Read the model definition and answer for the solid it produces. Units are mm, in the model's axes. A direction names the side the tool comes from. Give positions to 0.01 mm unless a question says otherwise; leave off trailing zeros. Loops run counter-clockwise (first coordinate to the right, second up) from the corner with the lowest first, then second, coordinate; pieces in that order, holes last. Notation, with made-up numbers: (53.25, 89.5) -> (112.25, 89.5) arc R24 cw to (112.25, 119.5) -> close; hole circle Ø5 at (21.25, 41). An arc over 180 degrees is marked (long way). Return JSON: item names as keys, results as strings. Group by question number.
from build123d import *

# Parameters (mm, degrees)
SKETCH1_W               = 228.6
SKETCH1_H               = 228.6
BOSS_EXTRUDE1_DEPTH     = 67
SKETCH2_W               = 35.766
SKETCH2_H               = 35.766
CUT_EXTRUDE1_DEPTH      = 76.2
CUT_EXTRUDE3_DEPTH      = 4
CUT_EXTRUDE3_DEPTH_BACK = 4
SKETCH4_W               = 67
SKETCH4_H               = 35.766
CUT_EXTRUDE4_DEPTH      = 4
CUT_EXTRUDE4_DEPTH_BACK = 4
SKETCH5_W               = 67
SKETCH5_H               = 37.77
SKETCH5_H_2             = 35.766
CUT_EXTRUDE5_DEPTH      = 4
CUT_EXTRUDE5_DEPTH_BACK = 4
SKETCH6_W               = 67
SKETCH6_H               = 35.766
SKETCH6_H_2             = 37.77
CUT_EXTRUDE6_DEPTH      = 4
CUT_EXTRUDE6_DEPTH_BACK = 4
SKETCH9_W               = 67
SKETCH9_H               = 37.766
SKETCH9_H_2             = 35.766
SKETCH9_H_3             = 37.77
SKETCH10_W              = 67
SKETCH10_H              = 2
CUT_EXTRUDE7_DEPTH      = 233.316821509
SKETCH11_W              = 67
SKETCH11_H              = 2
CUT_EXTRUDE8_DEPTH      = 231.673489808


with BuildPart() as part:
    # Sketch1 → Boss-Extrude1 (new body)
    with BuildSketch(Plane(origin=(0, 0, 0), x_dir=(0, 0, -1), z_dir=(1, 0, 0))):
        Rectangle(SKETCH1_W, SKETCH1_H)
    extrude(amount=BOSS_EXTRUDE1_DEPTH)

    # Sketch2 → Cut-Extrude1 (cut)
    with BuildSketch(Plane(origin=(67, 0, 0), x_dir=(0, 0, -1), z_dir=(1, 0, 0))):
        with Locations((-94.417, 94.417)):
            Rectangle(SKETCH2_W, SKETCH2_H)
        with Locations((-56.651, 94.417)):
            Rectangle(SKETCH2_W, SKETCH2_H)
        with Locations((18.881, 94.417)):
            Rectangle(SKETCH2_W, SKETCH2_H)
        with Locations((-18.885, 94.417)):
            Rectangle(SKETCH2_W, SKETCH2_H)
        with Locations((56.647, 94.417)):
            Rectangle(SKETCH2_W, SKETCH2_H)
        with Locations((94.413, 94.417)):
            Rectangle(SKETCH2_W, SKETCH2_H)
        with Locations((56.647, 56.651)):
            Rectangle(SKETCH2_W, SKETCH2_H)
        with Locations((94.413, 56.651)):
            Rectangle(SKETCH2_W, SKETCH2_H)
        with Locations((18.881, 56.651)):
            Rectangle(SKETCH2_W, SKETCH2_H)
        with Locations((-18.885, 56.651)):
            Rectangle(SKETCH2_W, SKETCH2_H)
        with Locations((-56.651, 56.651)):
            Rectangle(SKETCH2_W, SKETCH2_H)
        with Locations((-94.417, 56.651)):
            Rectangle(SKETCH2_W, SKETCH2_H)
        with Locations((-94.417, 18.885)):
            Rectangle(SKETCH2_W, SKETCH2_H)
        with Locations((-56.651, 18.885)):
            Rectangle(SKETCH2_W, SKETCH2_H)
        with Locations((-18.885, 18.885)):
            Rectangle(SKETCH2_W, SKETCH2_H)
        with Locations((18.881, 18.885)):
            Rectangle(SKETCH2_W, SKETCH2_H)
        with Locations((56.647, 18.885)):
            Rectangle(SKETCH2_W, SKETCH2_H)
        with Locations((94.413, 18.885)):
            Rectangle(SKETCH2_W, SKETCH2_H)
        with Locations((94.413, -18.881)):
            Rectangle(SKETCH2_W, SKETCH2_H)
        with Locations((56.647, -18.881)):
            Rectangle(SKETCH2_W, SKETCH2_H)
        with Locations((18.881, -18.881)):
            Rectangle(SKETCH2_W, SKETCH2_H)
        with Locations((-18.885, -18.881)):
            Rectangle(SKETCH2_W, SKETCH2_H)
        with Locations((-56.651, -18.881)):
            Rectangle(SKETCH2_W, SKETCH2_H)
        with Locations((-94.417, -18.881)):
            Rectangle(SKETCH2_W, SKETCH2_H)
        with Locations((56.647, -56.647)):
            Rectangle(SKETCH2_W, SKETCH2_H)
        with Locations((94.413, -56.647)):
            Rectangle(SKETCH2_W, SKETCH2_H)
        with Locations((94.413, -94.413)):
            Rectangle(SKETCH2_W, SKETCH2_H)
        with Locations((56.647, -94.413)):
            Rectangle(SKETCH2_W, SKETCH2_H)
        with Locations((18.881, -94.413)):
            Rectangle(SKETCH2_W, SKETCH2_H)
        with Locations((18.881, -56.647)):
            Rectangle(SKETCH2_W, SKETCH2_H)
        with Locations((-18.885, -56.647)):
            Rectangle(SKETCH2_W, SKETCH2_H)
        with Locations((-18.885, -94.413)):
            Rectangle(SKETCH2_W, SKETCH2_H)
        with Locations((-56.651, -94.413)):
            Rectangle(SKETCH2_W, SKETCH2_H)
        with Locations((-56.651, -56.647)):
            Rectangle(SKETCH2_W, SKETCH2_H)
        with Locations((-94.417, -94.413)):
            Rectangle(SKETCH2_W, SKETCH2_H)
        with Locations((-94.417, -56.647)):
            Rectangle(SKETCH2_W, SKETCH2_H)
    extrude(amount=-CUT_EXTRUDE1_DEPTH, mode=Mode.SUBTRACT)

    # Sketch4 → Cut-Extrude3 (cut, two sides: drawn at the far end of the back side and taken through both)
    with BuildSketch(Plane(origin=(0, -114.3, 0), x_dir=(1, 0, 0), z_dir=(0, 1, 0)).offset(-CUT_EXTRUDE3_DEPTH_BACK)):
        with Locations((33.5, -94.417)):
            Rectangle(SKETCH4_W, SKETCH4_H)
        with Locations((33.5, -56.651)):
            Rectangle(SKETCH4_W, SKETCH4_H)
        with Locations((33.5, -18.885)):
            Rectangle(SKETCH4_W, SKETCH4_H)
        with Locations((33.5, 18.881)):
            Rectangle(SKETCH4_W, SKETCH4_H)
        with Locations((33.5, 56.647)):
            Rectangle(SKETCH4_W, SKETCH4_H)
        with Locations((33.5, 94.413)):
            Rectangle(SKETCH4_W, SKETCH4_H)
    extrude(amount=CUT_EXTRUDE3_DEPTH + CUT_EXTRUDE3_DEPTH_BACK, mode=Mode.SUBTRACT)

    # Sketch5 → Cut-Extrude4 (cut, two sides: drawn at the far end of the back side and taken through both)
    with BuildSketch(Plane.XY.offset(114.3).offset(-CUT_EXTRUDE4_DEPTH_BACK)):
        with Locations((33.5, -95.415)):
            Rectangle(SKETCH5_W, SKETCH5_H)
        with Locations((33.5, -56.647)):
            Rectangle(SKETCH5_W, SKETCH5_H_2)
        with Locations((33.5, -18.881)):
            Rectangle(SKETCH5_W, SKETCH5_H_2)
        with Locations((33.5, 18.885)):
            Rectangle(SKETCH5_W, SKETCH5_H_2)
        with Locations((33.5, 56.651)):
            Rectangle(SKETCH5_W, SKETCH5_H_2)
        with Locations((33.5, 94.417)):
            Rectangle(SKETCH5_W, SKETCH5_H_2)
    extrude(amount=CUT_EXTRUDE4_DEPTH + CUT_EXTRUDE4_DEPTH_BACK, mode=Mode.SUBTRACT)

    # Sketch6 → Cut-Extrude5 (cut, two sides: drawn at the far end of the back side and taken through both)
    with BuildSketch(Plane.XY.offset(-114.3).offset(-CUT_EXTRUDE5_DEPTH_BACK)):
        with Locations((33.5, 94.417)):
            Rectangle(SKETCH6_W, SKETCH6_H)
        with Locations((33.5, 56.651)):
            Rectangle(SKETCH6_W, SKETCH6_H)
        with Locations((33.5, 18.885)):
            Rectangle(SKETCH6_W, SKETCH6_H)
        with Locations((33.5, -18.881)):
            Rectangle(SKETCH6_W, SKETCH6_H)
        with Locations((33.5, -56.647)):
            Rectangle(SKETCH6_W, SKETCH6_H)
        with Locations((33.5, -95.415)):
            Rectangle(SKETCH6_W, SKETCH6_H_2)
    extrude(amount=CUT_EXTRUDE5_DEPTH + CUT_EXTRUDE5_DEPTH_BACK, mode=Mode.SUBTRACT)

    # Sketch9 → Cut-Extrude6 (cut, two sides: drawn at the far end of the back side and taken through both)
    with BuildSketch(Plane(origin=(0, 114.3, 0), x_dir=(1, 0, 0), z_dir=(0, 1, 0)).offset(-CUT_EXTRUDE6_DEPTH_BACK)):
        with Locations((33.5, -95.417)):
            Rectangle(SKETCH9_W, SKETCH9_H)
        with Locations((33.5, -56.651)):
            Rectangle(SKETCH9_W, SKETCH9_H_2)
        with Locations((33.5, -18.885)):
            Rectangle(SKETCH9_W, SKETCH9_H_2)
        with Locations((33.5, 18.881)):
            Rectangle(SKETCH9_W, SKETCH9_H_2)
        with Locations((33.5, 56.647)):
            Rectangle(SKETCH9_W, SKETCH9_H_2)
        with Locations((33.5, 95.415)):
            Rectangle(SKETCH9_W, SKETCH9_H_3)
    extrude(amount=CUT_EXTRUDE6_DEPTH + CUT_EXTRUDE6_DEPTH_BACK, mode=Mode.SUBTRACT)

    # Sketch10 → Cut-Extrude7 (cut, through all)
    with BuildSketch(Plane.XY.offset(76.534)):
        with Locations((33.5, -113.3)):
            Rectangle(SKETCH10_W, SKETCH10_H)
        with Locations((33.5, 113.3)):
            Rectangle(SKETCH10_W, SKETCH10_H)
    extrude(amount=-CUT_EXTRUDE7_DEPTH, mode=Mode.SUBTRACT)

    # Sketch11 → Cut-Extrude8 (cut, through all)
    with BuildSketch(Plane(origin=(0, -76.53, 0), x_dir=(-1, 0, 0), z_dir=(0, -1, 0))):
        with Locations((-33.5, 113.3)):
            Rectangle(SKETCH11_W, SKETCH11_H)
        with Locations((-33.5, -113.3)):
            Rectangle(SKETCH11_W, SKETCH11_H)
    extrude(amount=-CUT_EXTRUDE8_DEPTH, mode=Mode.SUBTRACT)


solid = part.part
1. A straight line is drawn through the part: line 1 (Y direction, x = 20, z = 18.5). Find the intervals that lie inside material, in ascending order. Write a range as from..to.
2. Which of the six approach directions +Z, -Z, +X, -X, +Y, -Y give full straight-line access (tool end or side, diameter ignored) to faces 5 (the flat face through (33, -95, -36.764)), 6 (the flat face through (34, -0.998, 95)), 7 (the flat face through (34, 36.768, -19))?
3. Section C-C on x = 11 is taken. State how many separate pieces and enclosed holes the cut face has, then the cut area to 3 significant figures.
4. Flat-ended cylindrical pins translate along their axes: pin 1 Ø6 at (x, y) = (36.5, -10) entering from -Z; pin 2 Ø18 at (x, z) = (21, -64.5) entering from -Y; pin 3 Ø10.5 at (x, z) = (24.5, 98) entering from +Y. Find the tip coordinate at first contact, or state that the pin passes through.
5. Section A-A on z = 24.5 is taken. Determine the outline of the cut face in (x, y), then the cut area to 3 significant figures.
6. Determine the mould class of faces 1 (the flat face through (33, 94, -76.53)), 2 (the flat face through (34, 74.534, 19)), 3 (the flat face through (33, -95, 1.002)), 4 (the flat face through (33, 38.768, 94)) for opening direction Z: pulls with the +Z half, pulls with the -Z half, needs draft (parallel to the pull), parting line crosses it, or undercut.
Completed:
{
 "1": {"line 1": "y = -76.53..-74.53, -38.76..-36.76, -1..1, 36.77..38.77, 74.53..76.53"},
 "2": {"face 5": "+X, -X, -Y", "face 6": "+Z, +X, -X", "face 7": "+X, -X"},
 "3": {"separate pieces": "1", "enclosed holes": "16", "area": "4,390 mm²"},
 "4": {"pin 1": "stops at z = -76.53", "pin 2": "stops at y = -76.53", "pin 3": "stops at y = 76.53"},
 "5": {"outline": "(0, -76.53) -> (67, -76.53) -> (67, -74.53) -> (0, -74.53) -> close; (0, -38.76) -> (67, -38.76) -> (67, -36.76) -> (0, -36.76) -> close; (0, -1) -> (67, -1) -> (67, 1) -> (0, 1) -> close; (0, 36.77) -> (67, 36.77) -> (67, 38.77) -> (0, 38.77) -> close; (0, 74.53) -> (67, 74.53) -> (67, 76.53) -> (0, 76.53) -> close", "area": "670 mm²"},
 "6": {"face 1": "pulls with the -Z half", "face 2": "undercut", "face 3": "undercut", "face 4": "needs draft"}
}
